Geometry check sheet. Reference: the model listing, model coordinates, mm. A direction names the side the tool comes from. Give positions to 0.01 mm unless a question says otherwise; leave off trailing zeros. Loops run counter-clockwise (first coordinate to the right, second up) from the corner with the lowest first, then second, coordinate; pieces in that order, holes last. Notation, with made-up numbers: (7, -12) -> (43, -12) arc R28 ccw to (43, 15) -> close; hole circle Ø9 at (57, -21). An arc over 180 degrees is marked (long way). One line per item, written item: value. Start each with the question number.
(1) Sectioned sample at A-A, the plane z = 0. State how many separate pieces and enclosed holes the cut face has, then the cut area to 3 significant figures.
(2) Scan lines: line 1 along Z through (x, y) = (240, 259); line 2 along Z through (x, y) = (270, 248); line 3 along Y through (x, z) = (15, 0). Record each from-to range of solid material in increasing order. Write a range as from..to.
(3) Draft check along X on faces 5 (the face through (10.14, -4.868, 66.349)), 6 (the face through (0, -16, 32)), 7 (the face through (20, -16, 49)). Enter one of: pulls with the +X half, pulls with the -X half, needs draft (parallel to the pull), parting line crosses it, or undercut.
(4) Gauge pin test, flat ends, axial feed: pin 1 Ø9.5 at (y, z) = (0, -60) entering from -X; pin 2 Ø18.5 at (y, z) = (-51.96, 30) entering from +X; pin 3 Ø10 at (x, z) = (175.5, 46) entering from -Y; pin 4 Ø6 at (x, z) = (189.5, -1) entering from -Y. Record the tip position at first contact, or that the pin passes through.
(5) Tool access check on faces 1 (the face through (307.63, 259.86, 49.56)), 2 (the face through (9.86, 50.92, 37.93)), 3 (the face through (254.98, 225.35, -47.69)), 4 (the face through (202, 260, 0)). Record the directions out of +Z, -Z, +X, -X, +Y, -Y that give a thin tool (end or side, any length) a straight path to the whole face; none if there is none.
(6) Sectioned sample at D-D, the plane y = 234. Record the cut outline in (x, z).
from build123d import *

# Parameters (mm, degrees)
SKETCH2_R             = 50
SKETCH2_R_2           = 35
SKETCH3_R             = 75
SKETCH3_R_2           = 35
BOSS_EXTRUDE1_DEPTH   = 20
BOSS_EXTRUDE2_START   = -20
SKETCH4_R             = 75
SKETCH4_R_2           = 35
BOSS_EXTRUDE2_DEPTH   = 20
HOLE1_D               = 16
CIRPATTERN1_OUTLINE_R = 8
CIRPATTERN1_DEPTH     = 20
HOLE2_D               = 16
CIRPATTERN2_START     = 250
CIRPATTERN2_OUTLINE_R = 8
CIRPATTERN2_DEPTH     = 20


# Read off the part's stored shape, not the designer's step: CirPattern1, CirPattern2
with BuildPart() as part:
    # Sweep1: sweep along a path in Sketch1
    with BuildLine(Plane.XY) as sweep1_path:
        Line((0, 0), (70, 0))
        ThreePointArc((70, 0), (211.421356237, 58.578643763), (270, 200))
        Line((270, 200), (270, 270))
    # Sketch2 → Sweep1 (sweep)
    with BuildSketch(Plane(origin=(0, 0, 0), x_dir=(0, 0, -1), z_dir=(1, 0, 0))):
        Circle(SKETCH2_R)
        Circle(SKETCH2_R_2, mode=Mode.SUBTRACT)
    sweep(path=sweep1_path.line)

    # Sketch3 → Boss-Extrude1 (add)
    with BuildSketch(Plane(origin=(0, 270, 0), x_dir=(1, 0, 0), z_dir=(0, 1, 0))):
        with Locations(Location((270, 0, 0), (0, 0, 270))):
            Circle(SKETCH3_R)
        with Locations((270, 0)):
            Circle(SKETCH3_R_2, mode=Mode.SUBTRACT)
    extrude(amount=-BOSS_EXTRUDE1_DEPTH)

    # Sketch4 → Boss-Extrude2 (add)
    with BuildSketch(Plane.ZY.offset(BOSS_EXTRUDE2_START)):
        Circle(SKETCH4_R)
        with Locations(Location((0, 0, 0), (0, 0, 180))):
            Circle(SKETCH4_R_2, mode=Mode.SUBTRACT)
    extrude(amount=BOSS_EXTRUDE2_DEPTH)

    # Hole1 (through all)
    with Locations(Plane.ZY):
        with Locations((60, 0)):
            Hole(HOLE1_D / 2)

    # CirPattern1 outline → CirPattern1 (cut)
    with BuildSketch(Plane.YZ):
        with Locations((51.961524227, 30)):
            Circle(CIRPATTERN1_OUTLINE_R)
        with Locations((51.961524227, -30)):
            Circle(CIRPATTERN1_OUTLINE_R)
        with Locations((0, -60)):
            Circle(CIRPATTERN1_OUTLINE_R)
        with Locations((-51.961524227, -30)):
            Circle(CIRPATTERN1_OUTLINE_R)
        with Locations((-51.961524227, 30)):
            Circle(CIRPATTERN1_OUTLINE_R)
    extrude(amount=CIRPATTERN1_DEPTH, mode=Mode.SUBTRACT)

    # Hole2 (through all)
    with Locations(Plane(origin=(0, 270, 0), x_dir=(1, 0, 0), z_dir=(0, 1, 0))):
        with Locations((330, 0)):
            Hole(HOLE2_D / 2)

    # CirPattern2 outline → CirPattern2 (cut)
    with BuildSketch(Plane(origin=(0, 0, 0), x_dir=(1, 0, 0), z_dir=(0, 1, 0)).offset(CIRPATTERN2_START)):
        with Locations((300, -51.961524227)):
            Circle(CIRPATTERN2_OUTLINE_R)
        with Locations((240, -51.961524227)):
            Circle(CIRPATTERN2_OUTLINE_R)
        with Locations((210, 0)):
            Circle(CIRPATTERN2_OUTLINE_R)
        with Locations((240, 51.961524227)):
            Circle(CIRPATTERN2_OUTLINE_R)
        with Locations((300, 51.961524227)):
            Circle(CIRPATTERN2_OUTLINE_R)
    extrude(amount=CIRPATTERN2_DEPTH, mode=Mode.SUBTRACT)


solid = part.part
Calculated:
1. separate pieces: 4
1. enclosed holes: 0
1. area: 15,000 mm2
2. line 1: z = -68.74..-59.96, -43.96..-18.03, 18.03..43.96, 59.96..68.74
2. line 2: z = -50..-35, 35..50
2. line 3: y = -75..-35, 35..75
3. face 5: needs draft
3. face 6: pulls with the -X half
3. face 7: undercut
4. pin 1: passes through
4. pin 2: stops at x = 20
4. pin 3: stops at y = -3.22
4. pin 4: stops at y = -21.19
5. face 1: +Y, -Y
5. face 2: -X
5. face 3: none
5. face 4: +Y
6. outline: circle Ø100 at (270, 0); hole circle Ø70 at (270, 0)
